For this review, take the finished solid that the model builds, in its own axes (mm). A direction names the side the tool comes from. Round coordinates to 2 decimals unless told otherwise and drop trailing zeros. Order: outer loops, then holes, each group sorted by start corner. A loop starts at its lowest first (then second) coordinate and runs counter-clockwise, first axis right, second up. Notation, with made-up numbers: M 44,-37.5 L 72,-37.5 A7 cw 72,-32.5 Z; hole C -26.75,63.25 d6. An arc over 180 degrees is marked long. Use a Markdown table: item, result.
from build123d import *

# Parameters (mm, degrees)
SKETCH1_W           = 13
SKETCH1_H           = 33
BOSS_EXTRUDE1_DEPTH = 6
SKETCH2_R           = 4
BOSS_EXTRUDE2_DEPTH = 29.05598176
CUT_EXTRUDE1_REACH  = 41.286
SKETCH3_R           = 1
FILLET1_R           = 4


with BuildPart() as part:
    # Sketch1 → Boss-Extrude1 (new body)
    with BuildSketch(Plane.XY):
        Rectangle(SKETCH1_W, SKETCH1_H)
    extrude(amount=BOSS_EXTRUDE1_DEPTH)

    # Sketch2 → Boss-Extrude2 (add)
    with BuildSketch(Plane(origin=(0, 0, 0), x_dir=(-1, 0, 0), z_dir=(0, 0, -1))):
        Circle(SKETCH2_R)
    extrude(amount=BOSS_EXTRUDE2_DEPTH)

    # Sketch3 → Cut-Extrude1 (cut, up to next)
    with BuildSketch(Plane.XY.offset(6), mode=Mode.PRIVATE) as cut_extrude1_sk1:
        with Locations((0, 11)):
            Circle(SKETCH3_R)
    cut_extrude1_tool1 = extrude(cut_extrude1_sk1.sketch, amount=-CUT_EXTRUDE1_REACH, mode=Mode.PRIVATE) & part.part
    # Sketch3 → Cut-Extrude1 (cut, up to next)
    with BuildSketch(Plane.XY.offset(6), mode=Mode.PRIVATE) as cut_extrude1_sk2:
        with Locations((0, -11)):
            Circle(SKETCH3_R)
    cut_extrude1_tool2 = extrude(cut_extrude1_sk2.sketch, amount=-CUT_EXTRUDE1_REACH, mode=Mode.PRIVATE) & part.part
    add(cut_extrude1_tool1.solids().sort_by_distance((0, 11, 6))[0], mode=Mode.SUBTRACT)
    add(cut_extrude1_tool2.solids().sort_by_distance((0, -11, 6))[0], mode=Mode.SUBTRACT)

    # Fillet1
    fillet1_edges = [part.edges().sort_by_distance(p)[0] for p in [
        (6.5, 0, 6),
        (0, 16.5, 6),
        (-6.5, 0, 6),
        (0, -16.5, 6),
    ]]
    fillet(fillet1_edges, radius=FILLET1_R)


solid = part.part
Q1. Add section B-B (y = 0). Write out the cut boundary in (x, z), then the cut area to 3 significant figures.
Determined:
| item | result |
|---|---|
| outline | M -6.5,0 L -4,0 L -4,-29.06 L 4,-29.06 L 4,0 L 6.5,0 L 6.5,2 A4 ccw 2.5,6 L -2.5,6 A4 ccw -6.5,2 Z |
| area | 304 mm^2 |
Q2. Add section D-D (x = -3.5). Write out the cut boundary in (y, z).
Determined:
| item | result |
|---|---|
| outline | M -16.5,0 L -1.94,0 L -1.94,-29.06 L 1.94,-29.06 L 1.94,0 L 16.5,0 L 16.5,2 A4 ccw 13.5,5.87 L -13.5,5.87 A4 ccw -16.5,2 Z |
Q3. Wall thickness on line 1 along Y through (x, z) = (0, 1.2); line 2 along Y through (x, z) = (0, 2.7); line 3 along Z through (x, y) = (1, 4): over which ranges is each line inside the solid? List them lowest first. Write a range as [from, to].
Determined:
| item | result |
|---|---|
| line 1 | y = [-16.5, -12], [-10, 10], [12, 16.5] |
| line 2 | y = [-16.44, -12], [-10, 10], [12, 16.44] |
| line 3 | z = [0, 6] |
Q4. Machinability: for faces 1 (the cylindrical face through (0.867, -3.905, -14.325)), 2 (the flat face through (0, 0, 6)), which of the approach directions +Z, -Z, +X, -X, +Y, -Y give a long, thin tool a straight path to every point of the face, cutting with its end or side? Answer none if there is none.
Determined:
| item | result |
|---|---|
| face 1 | -Z |
| face 2 | +Z, +X, -X, +Y, -Y |
Q5. Add section A-A (x = 0). Write out the cut boundary in (y, z).
Determined:
| item | result |
|---|---|
| outline | M -16.5,0 L -12,0 L -12,6 L -12.5,6 A4 ccw -16.5,2 Z; M -10,0 L -4,0 L -4,-29.06 L 4,-29.06 L 4,0 L 10,0 L 10,6 L -10,6 Z; M 12,0 L 16.5,0 L 16.5,2 A4 ccw 12.5,6 L 12,6 Z |
Q6. Clearance check with flat-ended pins moving along their axes: pin 1 (2.5 mm diameter, centred on x = 0, y = -11, fed in from -Z); pin 2 (2 mm diameter, centred on x = -4.5, z = -20.5, fed in from -Y); pin 3 (1 mm diameter, centred on x = 0.5, z = -6, fed in from +Y); pin 4 (8 mm diameter, centred on y = -11.5, z = -1, fed in from -X). State where each tip first meets the part, or that it passes through.
Determined:
| item | result |
|---|---|
| pin 1 | stops at z = 0 |
| pin 2 | stops at y = -1.94 |
| pin 3 | stops at y = 4 |
| pin 4 | stops at x = -6.5 |
Q7. Add section C-C (z = -15). Write out the cut boundary in (x, y).
Determined:
| item | result |
|---|---|
| outline | C 0,0 d8 |
